Source: CAD feature listing. Evaluate the final solid. Frame: model axes, mm. Round coordinates to 2 decimals unless told otherwise and drop trailing zeros. Use a Markdown table: item, result.
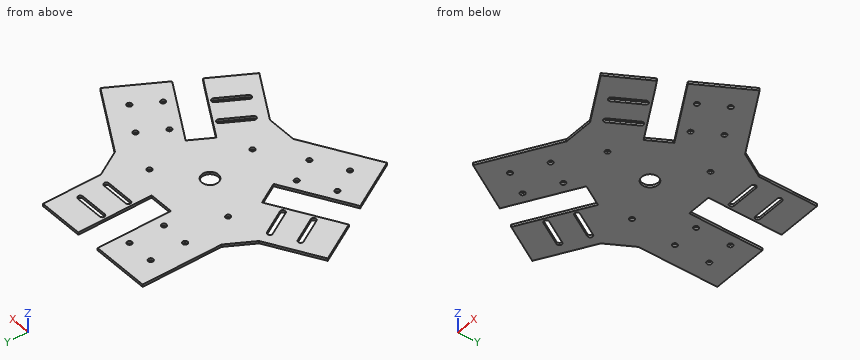
Autodesk Fusion 360 part; units mm, degrees
sketch "Boceto1" plane through (0, 0, 0) normal (0, 0, 1) x (1, 0, 0)
  circle A0 centre (0, 0) radius 100
  line L0 (0, 200.0885) -> (-173.2817, -100.0442)
  line L1 (-173.2817, -100.0442) -> (173.2817, -100.0442)
  line L2 (173.2817, -100.0442) -> (0, 200.0885)
  line L3 (0, -100.0442) -> (0, 200.0885) construction
  line L4 (-173.2817, -100.0442) -> (86.6408, 50.0221) construction
  line L5 (173.2817, -100.0442) -> (-86.6408, 50.0221) construction
  line L6 (51.9615, -30) -> (59.4615, -17.0096)
  line L7 (59.4615, -17.0096) -> (128.7436, -57.0096)
  line L8 (44.4615, -42.9904) -> (113.7436, -82.9904)
  line L9 (51.9615, -30) -> (44.4615, -42.9904)
  line L10 (-15, 60) -> (-15, 140)
  line L11 (0.5917, 60) -> (15, 60)
  line L12 (15, 60) -> (15, 140)
  line L13 (-123.1844, 140) -> (49.0279, 140)
  line L14 (-15, 60) -> (0.5917, 60)
  line L15 (157.2934, 41.8591) -> (75.3655, -100.0442)
  line L16 (-44.4615, -42.9904) -> (-113.7436, -82.9904)
  line L17 (-59.4615, -17.0096) -> (-128.7436, -57.0096)
  line L18 (-30.9577, -176.4773) -> (-124.184, -15.0046)
  line L19 (-44.4615, -42.9904) -> (-59.4615, -17.0096)
  circle A1 centre (0, 0) radius 10
  line L20 (-115.5498, 0.1381) -> (-24.8334, -156.9872) construction
  line L21 (212.8999, -69.8468) -> (210.5798, -60.2903) construction
  line L22 (57.7095, -100.0442) -> (164.8904, 85.5986) construction
  line L23 (57.7861, 100) -> (-125, 100) construction
  line L24 (-85, 150) -> (-15, 150)
  line L25 (-15, 150) -> (-15, 50)
  line L26 (-15, 50) -> (-85, 50)
  line L27 (-85, 50) -> (-85, 150)
  circle A2 centre (45, 84) radius 3
  circle A3 centre (25, 84) radius 3
  circle A4 centre (25, 116) radius 3
  circle A5 centre (45, 116) radius 3
  line L28 (28.8663, 150.0905) -> (70, 150.0905)
  line L29 (70, 150.0905) -> (70, 78.8449)
  line L30 (21, 113) -> (55, 113)
  line L31 (21, 119) -> (55, 119)
  arc A6 (55, 113) -> (55, 119) centre (55, 116) ccw
  arc A7 (21, 119) -> (21, 113) centre (21, 116) ccw
  line L32 (21, 81) -> (55, 81)
  circle A8 centre (25, 84) radius 3
  circle A9 centre (45, 84) radius 3
  line L33 (21, 87) -> (55, 87)
  arc A10 (21, 87) -> (21, 81) centre (21, 84) ccw
  arc A11 (55, 81) -> (55, 87) centre (55, 84) ccw
  line L34 (-0.8013, -98.6122) -> (-87.4038, -148.6122)
  line L35 (-35.8013, -37.9904) -> (-0.8013, -98.6122)
  line L36 (-44.4615, -42.9904) -> (-113.7436, -82.9904)
  line L37 (-122.4038, -87.9904) -> (-35.8013, -37.9904)
  line L38 (-87.4038, -148.6122) -> (-122.4038, -87.9904)
  line L39 (-59.6514, -176.6808) -> (-145.7575, -27.5406)
  line L40 (-59.4615, -17.0096) -> (-128.7436, -57.0096)
  line L41 (-52.2574, -29.4875) -> (-59.4615, -17.0096)
  line L42 (-44.4615, -42.9904) -> (-52.2574, -29.4875)
  line L43 (-80.6481, -22.3135) -> (-97.6481, 7.1314)
  circle A12 centre (-112.9589, -36.3494) radius 3
  circle A13 centre (-122.9589, -19.0289) radius 3
  circle A14 centre (-85.2461, -20.3494) radius 3
  circle A15 centre (-95.2461, -3.0289) radius 3
  line L44 (-85.8442, -25.3135) -> (-102.8442, 4.1314)
  arc A16 (-85.8442, -25.3135) -> (-80.6481, -22.3135) centre (-83.2461, -23.8135) ccw
  arc A17 (-97.6481, 7.1314) -> (-102.8442, 4.1314) centre (-100.2461, 5.6314) ccw
  arc A18 (-113.557, -41.3135) -> (-108.3609, -38.3135) centre (-110.9589, -39.8135) ccw
  line L45 (-108.3609, -38.3135) -> (-125.3609, -8.8686)
  line L46 (-113.557, -41.3135) -> (-130.557, -11.8686)
  arc A19 (-125.3609, -8.8686) -> (-130.557, -11.8686) centre (-127.9589, -10.3686) ccw
  line L47 (-144.4154, -50.0463) -> (-164.9822, -14.4235)
  line L48 (-164.9822, -14.4235) -> (-103.2817, 21.1993)
  line L49 (85.8013, 48.6122) -> (172.4038, -1.3878)
  line L50 (50.8013, -12.0096) -> (85.8013, 48.6122)
  line L51 (59.4615, -17.0096) -> (128.7436, -57.0096)
  line L52 (137.4038, -62.0096) -> (50.8013, -12.0096)
  line L53 (172.4038, -1.3878) -> (137.4038, -62.0096)
  line L54 (182.8357, 36.6808) -> (96.7296, -112.4594)
  line L55 (44.4615, -42.9904) -> (113.7436, -82.9904)
  line L56 (51.6657, -30.5125) -> (44.4615, -42.9904)
  line L57 (59.4615, -17.0096) -> (51.6657, -30.5125)
  line L58 (59.6481, -58.6865) -> (42.6481, -88.1314)
  circle A20 centre (87.9589, -79.6506) radius 3
  circle A21 centre (77.9589, -96.9711) radius 3
  circle A22 centre (60.2461, -63.6506) radius 3
  circle A23 centre (50.2461, -80.9711) radius 3
  line L59 (64.8442, -61.6865) -> (47.8442, -91.1314)
  arc A24 (64.8442, -61.6865) -> (59.6481, -58.6865) centre (62.2461, -60.1865) ccw
  arc A25 (42.6481, -88.1314) -> (47.8442, -91.1314) centre (45.2461, -89.6314) ccw
  arc A26 (92.557, -77.6865) -> (87.3609, -74.6865) centre (89.9589, -76.1865) ccw
  line L60 (87.3609, -74.6865) -> (70.3609, -104.1314)
  line L61 (92.557, -77.6865) -> (75.557, -107.1314)
  arc A27 (70.3609, -104.1314) -> (75.557, -107.1314) centre (72.9589, -105.6314) ccw
  line L62 (115.549, -100.0442) -> (94.9822, -135.667)
  line L63 (94.9822, -135.667) -> (33.2817, -100.0442)
  line L64 (-15, 150) -> (28.8663, 150.0905)
  line L65 (15, 150.0619) -> (15, 140)
  line L66 (-144.4154, -50.0463) -> (-122.4038, -87.9904)
  line L67 (115.549, -100.0442) -> (137.4038, -62.0096)
  line L68 (122.3417, -88.2227) -> (113.7436, -82.9904)
  line L69 (-137.4729, -62.0138) -> (-128.7436, -57.0096)
  circle A28 centre (118.8973, -36.3138) radius 3
  circle A29 centre (135.4123, -7.709) radius 3
  circle A30 centre (98.8228, 13.416) radius 3
  circle A31 centre (82.3078, -15.1888) radius 3
  circle A32 centre (-61.03, 121.125) radius 3
  circle A33 centre (-28, 121.125) radius 3
  circle A34 centre (-28, 78.875) radius 3
  circle A35 centre (-61.03, 78.875) radius 3
  circle A36 centre (-74.3823, -113.416) radius 3
  circle A37 centre (-90.8973, -84.8112) radius 3
  circle A38 centre (-54.3078, -63.6862) radius 3
  circle A39 centre (-37.7928, -92.291) radius 3
  line L70 (-3.1207, -99.9513) -> (33.2817, -100.0442)
  line L71 (-103.2817, 21.1993) -> (-85, 52.8641)
  line L72 (0, 0) -> (15.0803, -100.0442) construction
  circle A40 centre (8.9431, -59.3298) radius 3
  circle A41 centre (0, 0) radius 60 construction
  circle A42 centre (46.9095, 37.4099) radius 3
  circle A43 centre (-55.8526, 21.9199) radius 3
  point P0 (-86.6025, -50)
  point P1 (-85.2461, -20.3494)
  point P2 (60.2461, -63.6506)
  dimension "d1" = 200
  dimension "d5" = 80
  dimension "d6" = 60
  dimension "d7" = 30
  dimension "d8" = 80
  dimension "d9" = 30
  dimension "d10" = 15
  dimension "d13" = 60
  dimension "d16" = 80
  dimension "d17" = 30
  dimension "d18" = 15
  dimension "d19" = 60
  dimension "d22" = 80
  dimension "d24" = 80
  dimension "d25" = 20
  dimension "d27" = 70
  dimension "d28" = 100
  dimension "d29" = 50
  dimension "d47" = 6
  dimension "d48" = 6
  dimension "d49" = 6
  dimension "d50" = 6
  dimension "d51" = 20
  dimension "d52" = 20
  dimension "d53" = 32
  dimension "d55" = 10
  dimension "d56" = 10
  dimension "d57" = 16
  dimension "d58" = 16
  dimension "d59" = 32
  dimension "d60" = 10
  dimension "d61" = 4
  dimension "d62" = 4
  dimension "d63" = 10
  dimension "d68" = 6
  dimension "d69" = 13
  dimension "d70" = 21.125
  dimension "d71" = 6
  dimension "d72" = 33.03
  dimension "d73" = 21.125
  dimension "d74" = 21.125
  dimension "d76" = 360
  dimension "d94" = 36.4024
  dimension "d95" = 18.201
  dimension "d96" = 6
  dimension "d98" = 60
  dimension "d99" = 120
  dimension "d101" = 360
extrude "Extruir3" add sketch "Boceto1" along normal blind 3 contours A0 L7 L49 L50 L51 L52 A30 | A0 L2 L7 L15 L49 L51 L52 A30 | A0 L1 L8 L15 L55 L59 A25 A26 L60 L70 | A0 L6 L8 L9 L11 L12 L14 L17 L19 L25 L26 L27 L32 L33 A10 A11 L34 L35 L37 L40 L41 L42 L43 L44 A16 A17 L49 L50 L52 L55 L56 L57 L58 L59 A24 A25 L70 | L2 L7 L15 L51 L52 L54 | A0 L2 L12 L13 L30 L31 A7 L33 A11 L49 | L1 L8 L15 L54 L55 A26 L61 | L2 L52 L53 L54 | L2 L15 L49 L54 | L2 L15 L49 | L1 L54 L67 L68 | L2 L49 L53 L54 | L2 L28 L29 L30 L31 A6 | L1 L60 L61 A27 L62 L63 | A0 L1 L16 L18 L34 L36 L37 A39 | A0 L16 L34 L35 L36 L37 A39 | A0 L10 L25 L26 L27 A35 | A0 L0 L10 L13 L25 L27 A35 | L2 L13 L64 L65 | L1 L18 L34 | L0 L13 L24 L25 | L1 L18 L34 L39 | L1 L16 L18 L36 L37 L39 | L0 L13 L24 L27 | L0 L13 L27 | L1 L34 L38 L39 | L1 L37 L38 L39 | A0 L0 L17 L18 L27 L40 L44 A17 A18 L45 L71 | L0 L17 L18 L39 L40 A18 L46 | L0 L45 L46 A19 L47 L48 | L0 L39 L66 L69
Q1. Line query: L1, parallel to Y at x = 0, z = 1.05; L2, parallel to X at y = -114, z = 2.8; L3, parallel to X at y = -4, z = 2.1. Output: solid intervals per line, ascending.
Results are:
| item | result |
|---|---|
| L1 | -99.96 to -10, 10 to 60 |
| L2 | -107.39 to -77.32, -71.44 to -27.45, 57.45 to 107.49 |
| L3 | -146.93 to -98.15, -91.22 to -9.17, 9.17 to 170.9 |
Q2. Section A-A on z = 0.95. Give the number of separate pieces and of enclosed holes in the cut face, plus the area to 3 significant figures.
Results are:
| item | result |
|---|---|
| separate pieces | 1 |
| enclosed holes | 22 |
| area | 50,000 mm^2 |
Q3. First-contact query: pin 1 Ø0.9 at (y, z) = (93.5, 1.5) entering from -X; pin 2 Ø7 at (x, y) = (-54.31, -63.69) entering from -Z; pin 3 Ø3.5 at (x, y) = (-55.85, 21.92) entering from +Z; pin 4 Ø0.9 at (y, z) = (109, 1.5) entering from +X. Flat tips, straight axial feed; report the tip coordinate or a pass-through.
Results are:
| item | result |
|---|---|
| pin 1 | x = -85 |
| pin 2 | z = 0 |
| pin 3 | through |
| pin 4 | x = 70 |
